Here's how the part is built. I have some questions about the finished solid (model axes, mm). A direction names the side the tool comes from. Round coordinates to 2 decimals unless told otherwise and drop trailing zeros. Loops run counter-clockwise (first coordinate to the right, second up) from the corner with the lowest first, then second, coordinate; pieces in that order, holes last. Notation, with made-up numbers: M 66,33.25 L 74,33.25 A14 cw 74,45.25 Z; hole C 7.5,39.25 d5. An arc over 180 degrees is marked long. Use a Markdown table: item, result.
```python
from build123d import *

# Parameters (mm, degrees)
BOSS_EXTRUDE1_DEPTH    = 3.175
F_10_CLEARANCE_HOLE1_D = 5.1054
F_10_CLEARANCE_HOLE2_D = 5.1054
FILLET1_R              = 1.5875


with BuildPart() as part:
    # Sketch1 → Boss-Extrude1 (new body)
    with BuildSketch(Plane.XY):
        Polygon((0, 0), (0, 101.6), (-11.1125, 101.6), (-11.1125, 25.4), (-101.6, 25.4), (-101.6, 0), align=None)
    extrude(amount=BOSS_EXTRUDE1_DEPTH)

    # #10 Clearance Hole1 (through all)
    with Locations(Plane.XY.offset(3.175)):
        with Locations((-7.14375, 6.35), (-7.14375, 34.925), (-7.14375, 63.5), (-7.14375, 92.075)):
            Hole(F_10_CLEARANCE_HOLE1_D / 2)

    # #10 Clearance Hole2 (through all)
    with Locations(Plane.XY.offset(3.175)):
        with Locations((-88.9, 12.7), (-38.1, 12.7), (-63.5, 12.7)):
            Hole(F_10_CLEARANCE_HOLE2_D / 2)

    # Fillet1
    fillet1_edges = [part.edges().sort_by_distance(p)[0] for p in [
        (-101.6, 0, 1.5875),
        (-101.6, 25.4, 1.5875),
        (-11.1125, 101.6, 1.5875),
        (0, 101.6, 1.5875),
        (0, 0, 1.5875),
    ]]
    fillet(fillet1_edges, radius=FILLET1_R)


solid = part.part
```
Q1. I need wall thicknesses on line 1 (X direction, y = 15, z = 0.2); line 2 (Y direction, x = -38.1, z = 1.8); line 3 (Y direction, x = -56, z = 1.25). Which ranges of each line are inside material? Lowest first, please. Write a range as from..to.
Return value:
| item | result |
|---|---|
| line 1 | x = -101.6..-90.01, -87.79..-64.61, -62.39..-39.21, -36.99..0 |
| line 2 | y = 0..10.15, 15.25..25.4 |
| line 3 | y = 0..25.4 |
Q2. We'd pull the mould along Y, two halves only. Please class faces 1 (the cylindrical face through (-6.811, 37.456, 1.565)), 2 (the flat face through (-44, 25, 0)), 3 (the flat face through (-51, 0, 2)): pulls with the +Y half, pulls with the -Y half, needs draft (parallel to the pull), parting line crosses it, or undercut.
Return value:
| item | result |
|---|---|
| face 1 | undercut |
| face 2 | needs draft |
| face 3 | pulls with the -Y half |
Q3. Imagine slicing it at A-A, the plane y = 12.7. Please give me the cut outline in (x, z) (3 decimals).
Return value:
| item | result |
|---|---|
| outline | M -101.6,0 L -91.453,0 L -91.453,3.175 L -101.6,3.175 Z; M -86.347,0 L -66.053,0 L -66.053,3.175 L -86.347,3.175 Z; M -60.947,0 L -40.653,0 L -40.653,3.175 L -60.947,3.175 Z; M -35.547,0 L 0,0 L 0,3.175 L -35.547,3.175 Z |
Q4. Will these pins go through, and if not, where does the flat tip stop? P1, Ø3, axis at x = -7.14, y = 6.35, coming from the +Z side; P2, Ø1, axis at y = 61, z = 1.5, coming from the -X side; P3, Ø1.6, axis at x = -44, z = 2, coming from the +Y side.
Return value:
| item | result |
|---|---|
| P1 | passes through |
| P2 | stops at x = -11.11 |
| P3 | stops at y = 25.4 |
Q5. For faces 4 (the flat face through (-11.112, 63, 2)), 5 (the cylindrical face through (-6.59, 61.01, 1.57)), which set-ups out of +Z, -Z, +X, -X, +Y, -Y let a thin tool reach every point of the face, with its end or its side?
Return value:
| item | result |
|---|---|
| face 4 | +Z, -Z, -X, +Y |
| face 5 | +Z, -Z |
Q6. Imagine slicing it at B-B, the plane x = -38.1. Please give me the cut outline in (y, z) (3 decimals), then the cut area to 3 significant figures.
Return value:
| item | result |
|---|---|
| outline | M 0,0 L 10.147,0 L 10.147,3.175 L 0,3.175 Z; M 15.253,0 L 25.4,0 L 25.4,3.175 L 15.253,3.175 Z |
| area | 64.4 mm^2 |
Q7. Imagine slicing it at D-D, the plane z = 1. Give the number of separate pieces and of enclosed holes in the cut face, then the cut area to 3 significant figures.
Return value:
| item | result |
|---|---|
| separate pieces | 1 |
| enclosed holes | 7 |
| area | 3,280 mm^2 |
Q8. Imagine slicing it at C-C, the plane y = 63.5. Please give me the cut outline in (x, z) (1 decimal).
Return value:
| item | result |
|---|---|
| outline | M -11.1,0 L -9.7,0 L -9.7,3.2 L -11.1,3.2 Z; M -4.6,0 L 0,0 L 0,3.2 L -4.6,3.2 Z |
